For this review, take the finished solid that the model builds, in its own axes (mm). A direction names the side the tool comes from. Give positions to 0.01 mm unless a question says otherwise; leave off trailing zeros. Write each loop counter-clockwise with the first axis right and the second up, starting at its lowest first coordinate (ties: lowest second). Pieces come first, ordered by that corner, then holes. Notation, with made-up numbers: (-24.5, 76) -> (7.5, 76) arc R26 cw to (7.5, 95) -> close; hole circle Ø4 at (70.5, 47.5). An arc over 180 degrees is marked (long way). Return JSON: item names as keys, results as strings.
from build123d import *

# Parameters (mm, degrees)
SKETCH_2_R             = 7.94
EXTRUDE_1_DEPTH        = 7.875
EXTRUDE_1_2_DEPTH      = 7.875
EXTRUDE_2_DEPTH        = 3.43
PATTERN_LINEAR_1_COUNT = 2
PATTERN_LINEAR_1_PITCH = 29.29
EXTRUDE_3_DEPTH        = 45.995
EXTRUDE_3_DEPTH_BACK   = 16.705
SKETCH_4_R             = 3.97
CHAMFER_1_SIZE         = 0.686


with BuildPart() as part:
    # Sketch 2 → Extrude 1 (new, symmetric)
    with BuildSketch(Plane.XY):
        with Locations((12.7, 0)):
            Circle(SKETCH_2_R)
    extrude(amount=EXTRUDE_1_DEPTH, both=True)



with BuildPart() as body_2:
    # Sketch 2 → Extrude 1 2 (new, symmetric)
    with BuildSketch(Plane.XY):
        with Locations((-12.7, 0)):
            Circle(SKETCH_2_R)
    extrude(amount=EXTRUDE_1_2_DEPTH, both=True)


with BuildPart() as part_1:
    add(part.part)

    add(body_2.part)  # Extrude 2 merges body 2
    # Sketch 3 → Extrude 2 (add)
    with BuildSketch(Plane.XY.offset(7.875)):
        with BuildLine():
            ThreePointArc((-10.428153415, 11.849174574), (-24.765, 0), (-10.428153415, -11.849174574))
            ThreePointArc((-10.428153415, -11.849174574), (0, -10.8585), (10.428153415, -11.849174574))
            ThreePointArc((10.428153415, -11.849174574), (24.765, 0), (10.428153415, 11.849174574))
            ThreePointArc((10.428153415, 11.849174574), (0, 10.8585), (-10.428153415, 11.849174574))
        make_face()
    extrude_2 = extrude(amount=EXTRUDE_2_DEPTH)

    # Mirror 1: Extrude 2 across plane
    add(extrude_2.mirror(Plane.XY))


with BuildPart() as pattern_linear_1_1:
    # Pattern Linear 1: pattern copy
    add(part_1.part.moved(Location(Vector(0, 0, 1) * (1 * PATTERN_LINEAR_1_PITCH))))


with BuildPart() as part_2:
    add(part_1.part)

    add(pattern_linear_1_1.part)  # Extrude 3 merges Pattern Linear 1_1
    # Sketch 4 → Extrude 3 (add, two sides: drawn at the far end of the back side and taken through both)
    with BuildSketch(Plane.XY.offset(-EXTRUDE_3_DEPTH_BACK)):
        with Locations(Location((12.7, 0, 0), (0, 0, 180))):
            Circle(SKETCH_4_R)
        with Locations(Location((-12.7, 0, 0), (0, 0, 180))):
            Circle(SKETCH_4_R)
    extrude(amount=EXTRUDE_3_DEPTH + EXTRUDE_3_DEPTH_BACK)

    # Chamfer 1
    chamfer_1_edges = [part_2.edges().sort_by_distance(p)[0] for p in [
        (16.67, 0, -16.705),
        (16.67, 0, 45.995),
        (-8.73, 0, -16.705),
        (-8.73, 0, 45.995),
    ]]
    chamfer(chamfer_1_edges, length=CHAMFER_1_SIZE)


solid = part_2.part
1. For faces 1 (the cylindrical face through (-0.15, -10.86, 9.57)), 2 (the cylindrical face through (-9.77, -2.68, 14.6)), 3 (the cylindrical face through (-9.77, -2.68, 42.92)), 4 (the cylindrical face through (-9.77, -2.68, -13.69)), list the 3-axis set-ups (+Z, -Z, +X, -X, +Y, -Y) from which the entire face can be reached by the end or side of a thin tool; tool diameter is ignored.
Results found:
{"face 1": "+Z, -Z, -Y", "face 2": "none", "face 3": "+Z", "face 4": "-Z"}
2. Add section B-B, the plane x = -4. State the section outline as (y, z) points (3 decimals), plus the area to 3 significant figures.
Results found:
{"outline": "(-11.003, -11.305) -> (11.003, -11.305) -> (11.003, -7.875) -> (-11.003, -7.875) -> close; (-11.003, 7.875) -> (11.003, 7.875) -> (11.003, 11.305) -> (-11.003, 11.305) -> close; (-11.003, 17.985) -> (11.003, 17.985) -> (11.003, 21.415) -> (-11.003, 21.415) -> close; (-11.003, 37.165) -> (11.003, 37.165) -> (11.003, 40.595) -> (-11.003, 40.595) -> close", "area": "302 mm²"}
3. Add section A-A, the plane y = 7. Count the separate pieces of the cut face and the enclosed holes in it, plus the area to 3 significant figures.
Results found:
{"separate pieces": "2", "enclosed holes": "2", "area": "1,090 mm²"}
4. Add section C-C, the plane z = -2. State the section outline as (x, y) points, plus the area to 3 significant figures.
Results found:
{"outline": "circle Ø15.88 at (-12.7, 0); circle Ø15.88 at (12.7, 0)", "area": "396 mm²"}
5. To check wall thickness, follow probe 1 along Z at (x, y) = (-22, -4.5) (3 decimals); probe 2 along Z at (x, y) = (-20, 0.5) (3 decimals); probe 3 along X at (y, z) = (-2, 28). State the ranges of each line that lie inside material, in increasing order.
Results found:
{"probe 1": "z = -11.305 to -7.875, 7.875 to 11.305, 17.985 to 21.415, 37.165 to 40.595", "probe 2": "z = -11.305 to 11.305, 17.985 to 40.595", "probe 3": "x = -20.38 to -5.02, 5.02 to 20.38"}
6. The part is to be moulded in two halves that separate along X. For faces 5 (the cylindrical face through (-5.127, 2.385, 29.4)), 6 (the flat face through (13, 0, 45.995)), say which applies: +X half, -X half, draft (parallel to the pull), parting line (faces both ways), or undercut.
Results found:
{"face 5": "undercut", "face 6": "draft"}
7. For pin 1 (6 mm diameter, centred on x = -17, y = 2.5, fed in from -Z) (3 decimals); pin 2 (5 mm diameter, centred on y = 3, z = -8.5, fed in from +X); pin 3 (1.5 mm diameter, centred on x = 5.5, y = -7.5, fed in from +Z) (3 decimals); pin 4 (6 mm diameter, centred on y = -6.5, z = -8.5, fed in from -X), all flat-tipped, find the tip position at first contact; note any pin that passes through.
Results found:
{"pin 1": "stops at z = -16.705", "pin 2": "stops at x = 24.75", "pin 3": "stops at z = 40.595", "pin 4": "stops at x = -24.25"}
